```python
from build123d import *

# Parameters (mm, degrees)
F0_R     = 2.75
F0_R_2   = 1.2
F1_DEPTH = 3


with BuildPart() as f1:
    # F0 (on Top) → F1 (new body)
    with BuildSketch(Plane.XY):
        with BuildLine():
            Line((101, 8.5), (104, 11.5))
            Line((104, 11.5), (104.5, 12))
            Line((104.5, 12), (104, 12))
            ThreePointArc((104, 12), (101.87868, 11.12132), (101, 9))
            Line((101, 9), (101, 8.5))
        make_face()
        with BuildLine():
            Line((105, 11.5), (108, 8.5))
            Line((108, 8.5), (108, 9))
            ThreePointArc((108, 9), (107.12132, 11.12132), (105, 12))
            Line((105, 12), (104.5, 12))
            Line((104.5, 12), (105, 11.5))
        make_face()
        Polygon((104, 11.5), (105, 11.5), (104.5, 12), align=None)
        with BuildLine():
            Line((0, 34), (0, 0))
            Line((0, 0), (15, 0))
            ThreePointArc((15, 0), (16.414214, 0.585786), (17, 2))
            Line((17, 2), (17, 8.5))
            Line((17, 8.5), (17, 9))
            ThreePointArc((17, 9), (17.87868, 11.12132), (20, 12))
            Line((20, 12), (20.5, 12))
            Line((20.5, 12), (21, 12))
            ThreePointArc((21, 12), (23.12132, 11.12132), (24, 9))
            Line((24, 9), (24, 8.5))
            Line((24, 8.5), (24, 2))
            ThreePointArc((24, 2), (24.585786, 0.585786), (26, 0))
            Line((26, 0), (36, 0))
            ThreePointArc((36, 0), (37.414214, 0.585786), (38, 2))
            Line((38, 2), (38, 8.5))
            Line((38, 8.5), (38, 9))
            ThreePointArc((38, 9), (38.87868, 11.12132), (41, 12))
            Line((41, 12), (41.5, 12))
            Line((41.5, 12), (42, 12))
            ThreePointArc((42, 12), (44.12132, 11.12132), (45, 9))
            Line((45, 9), (45, 8.5))
            Line((45, 8.5), (45, 2))
            ThreePointArc((45, 2), (45.585786, 0.585786), (47, 0))
            Line((47, 0), (57, 0))
            ThreePointArc((57, 0), (58.414214, 0.585786), (59, 2))
            Line((59, 2), (59, 8.5))
            Line((59, 8.5), (59, 9))
            ThreePointArc((59, 9), (59.87868, 11.12132), (62, 12))
            Line((62, 12), (62.5, 12))
            Line((62.5, 12), (63, 12))
            ThreePointArc((63, 12), (65.12132, 11.12132), (66, 9))
            Line((66, 9), (66, 8.5))
            Line((66, 8.5), (66, 2))
            ThreePointArc((66, 2), (66.585786, 0.585786), (68, 0))
            Line((68, 0), (78, 0))
            ThreePointArc((78, 0), (79.414214, 0.585786), (80, 2))
            Line((80, 2), (80, 8.5))
            Line((80, 8.5), (80, 9))
            ThreePointArc((80, 9), (80.87868, 11.12132), (83, 12))
            Line((83, 12), (83.5, 12))
            Line((83.5, 12), (84, 12))
            ThreePointArc((84, 12), (86.12132, 11.12132), (87, 9))
            Line((87, 9), (87, 8.5))
            Line((87, 8.5), (87, 2))
            ThreePointArc((87, 2), (87.585786, 0.585786), (89, 0))
            Line((89, 0), (99, 0))
            ThreePointArc((99, 0), (100.414214, 0.585786), (101, 2))
            Line((101, 2), (101, 8.5))
            Line((101, 8.5), (101, 9))
            ThreePointArc((101, 9), (101.87868, 11.12132), (104, 12))
            Line((104, 12), (104.5, 12))
            Line((104.5, 12), (105, 12))
            ThreePointArc((105, 12), (107.12132, 11.12132), (108, 9))
            Line((108, 9), (108, 8.5))
            Line((108, 8.5), (108, 2))
            ThreePointArc((108, 2), (108.585786, 0.585786), (110, 0))
            Line((110, 0), (118, 0))
            ThreePointArc((118, 0), (119.414214, 0.585786), (120, 2))
            Line((120, 2), (120, 7.5))
            Line((120, 7.5), (120, 8))
            ThreePointArc((120, 8), (121.171573, 10.828427), (124, 12))
            Line((124, 12), (124.5, 12))
            Line((124.5, 12), (125, 12))
            ThreePointArc((125, 12), (127.828427, 10.828427), (129, 8))
            Line((129, 8), (129, 7.5))
            Line((129, 7.5), (129, 2))
            ThreePointArc((129, 2), (129.585786, 0.585786), (131, 0))
            Line((131, 0), (139, 0))
            ThreePointArc((139, 0), (140.414214, 0.585786), (141, 2))
            Line((141, 2), (141, 7.5))
            Line((141, 7.5), (141, 8))
            ThreePointArc((141, 8), (142.171573, 10.828427), (145, 12))
            Line((145, 12), (145.5, 12))
            Line((145.5, 12), (146, 12))
            ThreePointArc((146, 12), (148.828427, 10.828427), (150, 8))
            Line((150, 8), (150, 7.5))
            Line((150, 7.5), (150, 2))
            ThreePointArc((150, 2), (150.585786, 0.585786), (152, 0))
            Line((152, 0), (167, 0))
            Line((167, 0), (167, 34))
            Line((167, 34), (0, 34))
        make_face()
        with Locations((7, 6)):
            Circle(F0_R, mode=Mode.SUBTRACT)
        with Locations((160, 6)):
            Circle(F0_R, mode=Mode.SUBTRACT)
        with Locations((20.5, 18)):
            Circle(F0_R_2, mode=Mode.SUBTRACT)
        with Locations((41.5, 18)):
            Circle(F0_R_2, mode=Mode.SUBTRACT)
        with Locations((62.5, 18)):
            Circle(F0_R_2, mode=Mode.SUBTRACT)
        with Locations((37.5, 29)):
            Circle(F0_R, mode=Mode.SUBTRACT)
        with Locations((83.5, 18)):
            Circle(F0_R_2, mode=Mode.SUBTRACT)
        with Locations((104.5, 18)):
            Circle(F0_R_2, mode=Mode.SUBTRACT)
        with Locations((124.5, 18)):
            Circle(F0_R_2, mode=Mode.SUBTRACT)
        with Locations((145.5, 18)):
            Circle(F0_R_2, mode=Mode.SUBTRACT)
        with Locations((83.5, 29)):
            Circle(F0_R, mode=Mode.SUBTRACT)
        with Locations((129.5, 29)):
            Circle(F0_R, mode=Mode.SUBTRACT)
        with BuildLine():
            Line((146, 11.5), (150, 7.5))
            Line((150, 7.5), (150, 8))
            ThreePointArc((150, 8), (148.828427, 10.828427), (146, 12))
            Line((146, 12), (145.5, 12))
            Line((145.5, 12), (146, 11.5))
        make_face()
        Polygon((145, 11.5), (146, 11.5), (145.5, 12), align=None)
        with BuildLine():
            Line((145, 11.5), (145.5, 12))
            Line((145.5, 12), (145, 12))
            ThreePointArc((145, 12), (142.171573, 10.828427), (141, 8))
            Line((141, 8), (141, 7.5))
            Line((141, 7.5), (145, 11.5))
        make_face()
        with BuildLine():
            Line((125, 11.5), (129, 7.5))
            Line((129, 7.5), (129, 8))
            ThreePointArc((129, 8), (127.828427, 10.828427), (125, 12))
            Line((125, 12), (124.5, 12))
            Line((124.5, 12), (125, 11.5))
        make_face()
        Polygon((124, 11.5), (125, 11.5), (124.5, 12), align=None)
        with BuildLine():
            Line((124, 11.5), (124.5, 12))
            Line((124.5, 12), (124, 12))
            ThreePointArc((124, 12), (121.171573, 10.828427), (120, 8))
            Line((120, 8), (120, 7.5))
            Line((120, 7.5), (124, 11.5))
        make_face()
        with BuildLine():
            Line((84, 12), (83.5, 12))
            Line((83.5, 12), (84, 11.5))
            Line((84, 11.5), (87, 8.5))
            Line((87, 8.5), (87, 9))
            ThreePointArc((87, 9), (86.12132, 11.12132), (84, 12))
        make_face()
        Polygon((83.5, 12), (83, 11.5), (84, 11.5), align=None)
        with BuildLine():
            Line((80, 9), (80, 8.5))
            Line((80, 8.5), (83, 11.5))
            Line((83, 11.5), (83.5, 12))
            Line((83.5, 12), (83, 12))
            ThreePointArc((83, 12), (80.87868, 11.12132), (80, 9))
        make_face()
        with BuildLine():
            Line((63, 12), (62.5, 12))
            Line((62.5, 12), (63, 11.5))
            Line((63, 11.5), (66, 8.5))
            Line((66, 8.5), (66, 9))
            ThreePointArc((66, 9), (65.12132, 11.12132), (63, 12))
        make_face()
        Polygon((62.5, 12), (62, 11.5), (63, 11.5), align=None)
        with BuildLine():
            Line((59, 9), (59, 8.5))
            Line((59, 8.5), (62, 11.5))
            Line((62, 11.5), (62.5, 12))
            Line((62.5, 12), (62, 12))
            ThreePointArc((62, 12), (59.87868, 11.12132), (59, 9))
        make_face()
        with BuildLine():
            Line((42, 12), (41.5, 12))
            Line((41.5, 12), (42, 11.5))
            Line((42, 11.5), (45, 8.5))
            Line((45, 8.5), (45, 9))
            ThreePointArc((45, 9), (44.12132, 11.12132), (42, 12))
        make_face()
        Polygon((41.5, 12), (41, 11.5), (42, 11.5), align=None)
        with BuildLine():
            Line((38, 9), (38, 8.5))
            Line((38, 8.5), (41, 11.5))
            Line((41, 11.5), (41.5, 12))
            Line((41.5, 12), (41, 12))
            ThreePointArc((41, 12), (38.87868, 11.12132), (38, 9))
        make_face()
        with BuildLine():
            Line((21, 12), (20.5, 12))
            Line((20.5, 12), (21, 11.5))
            Line((21, 11.5), (24, 8.5))
            Line((24, 8.5), (24, 9))
            ThreePointArc((24, 9), (23.12132, 11.12132), (21, 12))
        make_face()
        Polygon((20.5, 12), (20, 11.5), (21, 11.5), align=None)
        with BuildLine():
            Line((17, 9), (17, 8.5))
            Line((17, 8.5), (20, 11.5))
            Line((20, 11.5), (20.5, 12))
            Line((20.5, 12), (20, 12))
            ThreePointArc((20, 12), (17.87868, 11.12132), (17, 9))
        make_face()
    extrude(amount=F1_DEPTH)


solid = f1.part
```
Input: part model. Units: mm. Frame: model coordinates. A direction names the side the tool comes from. Give positions to 0.01 mm unless a question says otherwise; leave off trailing zeros. Order: outer loops, then holes, each group sorted by start corner. A loop starts at its lowest first (then second) coordinate and runs counter-clockwise, first axis right, second up. Notation, with made-up numbers: M 43.5,48 L 96.5,48 A15 ccw 96.5,66 Z; hole C -18.75,68 d6. An arc over 180 degrees is marked long. Return JSON: item names as keys, results as strings.
Item 1: Access query for faces 3 (the flat face through (52, 0, 1)), 4 (the flat face through (122, 9.5, 1.5)). Directions: +Z, -Z, +X, -X, +Y, -Y. A direction counts if a zero-diameter tool reaches every point of the face in a straight line with its end or side. Return the directions, or none.
Solutions:
{"face 3": "+Z, -Z, +X, -X, -Y", "face 4": "+Z, -Z, -Y"}
Item 2: Cut plane B-B (y = 6). State how many separate pieces and enclosed holes the cut face has, then the cut area to 3 significant figures.
Solutions:
{"separate pieces": "10", "enclosed holes": "0", "area": "309 mm^2"}
Item 3: Pull-direction query (X, two-part tool) for faces 1 (the flat face through (60.5, 10, 1.5)), 2 (the flat face through (94, 0, 1)); classes: +X half, -X half, draft (parallel to the pull), parting line (faces both ways), or undercut.
Solutions:
{"face 1": "undercut", "face 2": "draft"}
Item 4: Cut plane A-A (y = 29). Return loops of the section in (x, z), then the cut area to 4 significant figures.
Solutions:
{"outline": "M 0,0 L 34.75,0 L 34.75,3 L 0,3 Z; M 40.25,0 L 80.75,0 L 80.75,3 L 40.25,3 Z; M 86.25,0 L 126.75,0 L 126.75,3 L 86.25,3 Z; M 132.25,0 L 167,0 L 167,3 L 132.25,3 Z", "area": "451.5 mm^2"}
Item 5: Ray query, probe 1 along Y at (x, z) = (7, 1.15); probe 2 along Y at (x, z) = (20.5, 1.2); probe 3 along X at (y, z) = (26.5, 1.4). Return the intervals inside material, ascending.
Solutions:
{"probe 1": "0 to 3.25, 8.75 to 34", "probe 2": "11.5 to 16.8, 19.2 to 34", "probe 3": "0 to 36.35, 38.65 to 82.35, 84.65 to 128.35, 130.65 to 167"}
Item 6: First-contact query: P1, Ø1.1, axis at x = 145.5, z = 1.5, coming from the -Y side. Flat tip, straight axial feed; report the tip coordinate or a pass-through.
Solutions:
{"P1": "y = 11.45"}
